```python
from build123d import *

# Parameters (mm, degrees)
SKETCH1_R           = 37.5
BOSS_EXTRUDE2_DEPTH = 24
FILLET1_R           = 4
SKETCH2_R           = 2
CUT_EXTRUDE1_DEPTH  = 24
SKETCH3_R           = 1.5
CUT_EXTRUDE3_DEPTH  = 25
CIRPATTERN1_COUNT   = 3


with BuildPart() as part:
    # Sketch1 → Boss-Extrude2 (new body)
    with BuildSketch(Plane.XY):
        Circle(SKETCH1_R)
    extrude(amount=BOSS_EXTRUDE2_DEPTH)

    # Fillet1
    fillet1_edges = [part.edges().sort_by_distance(p)[0] for p in [
        (-37.5, 0, 0),
        (-37.5, 0, 24),
    ]]
    fillet(fillet1_edges, radius=FILLET1_R)

    # Sketch2 → Cut-Extrude1 (cut)
    with BuildSketch(Plane.XY.offset(24)):
        Circle(SKETCH2_R)
    extrude(amount=-CUT_EXTRUDE1_DEPTH, mode=Mode.SUBTRACT)

    # Sketch3 → Cut-Extrude3 (cut, through all)
    with BuildSketch(Plane.XY.offset(24)):
        with Locations((0, -8.5)):
            Circle(SKETCH3_R)
    cut_extrude3 = extrude(amount=-CUT_EXTRUDE3_DEPTH, mode=Mode.SUBTRACT)

    # CirPattern1: Cut-Extrude3 ×3 about axis
    cirpattern1_axis = Axis((0, 0, 0), (0, 0, 1))
    for i in range(1, CIRPATTERN1_COUNT):
        add(cut_extrude3.rotate(cirpattern1_axis, i * 360 / CIRPATTERN1_COUNT), mode=Mode.SUBTRACT)


solid = part.part
```
Check sheet for the modelled part. Datum: model origin and axes. Units: mm. Give positions to 0.01 mm unless a question says otherwise; leave off trailing zeros. Write each loop counter-clockwise with the first axis right and the second up, starting at its lowest first coordinate (ties: lowest second). Pieces come first, ordered by that corner, then holes. Notation, with made-up numbers: (37.25, 86) - (76.25, 86) arc R35 ccw to (76.25, 119) - close; hole circle Ø8 at (43.25, 71). An arc over 180 degrees is marked (long way). Answer as a JSON object with one key per item and string values. Group by question number.
1) Depth check by flat-ended pin: P1, Ø1.5, axis at y = 5, z = 12, coming from the +X side; P2, Ø10, axis at y = 19.5, z = 15, coming from the -X side; P3, Ø4, axis at y = 9, z = 4.5, coming from the +X side. Enter the tip coordinate at first touch or a pass-through.
2) Thickness scan on probe 1 along Y at (x, z) = (0, 7.5); probe 2 along Y at (x, z) = (-0.5, 8.5); probe 3 along X at (y, z) = (-4, 22). Record the ranges inside material, lowest first. Write a range as from..to.
3) Sectioned sample at C-C (z = 9.5). Record the cut outline in (x, y).
4) Sectioned sample at B-B (x = 0). Record the cut outline in (y, z).
5) Sectioned sample at A-A (y = 0). Record the cut outline in (x, z), then the cut area to 3 significant figures.
6) Release check for a two-part mould opening along Y. For faces 1 (the face through (7, 0, 24)), 2 (the face through (-7.686, 2.786, 12.168)), 3 (the face through (-4.88, 37.18, 11.89)), 4 (the face through (8.75, 3.68, 12.17)) record: pulls with the +Y half, pulls with the -Y half, needs draft (parallel to the pull), parting line crosses it, or undercut.
Geometry results:
{
 "1": {"P1": "stops at x = 37.26", "P2": "stops at x = -34.58", "P3": "stops at x = 36.84"},
 "2": {"probe 1": "y = -37.5..-10, -7..-2, 2..37.5", "probe 2": "y = -37.5..-9.91, -7.09..-1.94, 1.94..37.5", "probe 3": "x = -36.75..36.75"},
 "3": {"outline": "circle Ø75 at (0, 0); hole circle Ø3 at (-7.36, 4.25); hole circle Ø4 at (0, 0); hole circle Ø3 at (0, -8.5); hole circle Ø3 at (7.36, 4.25)"},
 "4": {"outline": "(-37.5, 4) arc R4 ccw to (-33.5, 0) - (-10, 0) - (-10, 24) - (-33.5, 24) arc R4 ccw to (-37.5, 20) - close; (-7, 0) - (-2, 0) - (-2, 24) - (-7, 24) - close; (2, 0) - (33.5, 0) arc R4 ccw to (37.5, 4) - (37.5, 20) arc R4 ccw to (33.5, 24) - (2, 24) - close"},
 "5": {"outline": "(-37.5, 4) arc R4 ccw to (-33.5, 0) - (-2, 0) - (-2, 24) - (-33.5, 24) arc R4 ccw to (-37.5, 20) - close; (2, 0) - (33.5, 0) arc R4 ccw to (37.5, 4) - (37.5, 20) arc R4 ccw to (33.5, 24) - (2, 24) - close", "area": "1,690 mm^2"},
 "6": {"face 1": "needs draft", "face 2": "undercut", "face 3": "parting line crosses it", "face 4": "undercut"}
}
